Could you check a few things on this model? Use its own coordinates, in mm. A direction names the side the tool comes from. Coordinates: 2 decimals unless noted, no trailing zeros. Loops run counter-clockwise (first coordinate to the right, second up) from the corner with the lowest first, then second, coordinate; pieces in that order, holes last. Notation, with made-up numbers: M 2.25,72 L 9.25,72 A23 cw 9.25,92 Z; hole C 4,-29.5 d5. An arc over 180 degrees is marked long. Return JSON: item names as keys, results as strings. Group by question number.
from build123d import *

# Parameters (mm, degrees)
F0_W         = 64.9794517085
F0_H         = 80.3038775921
F1_DEPTH     = 44.704
F2_T         = -2.54
F3_R         = 24.241575959
F1_FACE1_W   = 44.704
F1_FACE1_H   = 80.3038775921
F4_DEPTH     = 10.668
F5_R         = 25.1594880742
F6_DEPTH     = 9.652
F7_W         = 6.6666891798
F7_H         = 7.7688368037
F8_DEPTH     = 37.846
F9_W         = 7.7688368037
F9_H         = 6.8424391291
F10_DEPTH    = 28.956
F11_W        = 7.8935802502
F11_H        = 7.7688368037
F12_DEPTH    = 25.4
F13_DEPTH    = 25.4
F15_DEPTH    = 34.798
F16_T1_DEPTH = 205.6075505485
F17_W        = 7.7688368037
F17_H        = 7.1335003994
F18_DEPTH    = 27.178


# Not quite as in the source:
# - a fillet or chamfer that OpenCascade refuses, or shapes differently, is made with other operations: its cross-section is extruded or revolved along the edge and cut away or added


with BuildPart() as f1:
    # F0 (on Front) → F1 (new body)
    with BuildSketch(Plane.XZ):
        with Locations((25.8230366744, -3.7049613893)):
            Rectangle(F0_W, F0_H)
    extrude(amount=F1_DEPTH)

    # F2
    f2_openings = [f1.faces().sort_by_distance(p)[0] for p in [
        (25.823037, -22.352, 36.446977),
        (25.823037, -44.704, -3.704961),
    ]]
    offset(amount=F2_T, openings=f2_openings)

    # F3 (on face) + F1_face1 (on face) → F4 (join)
    with BuildSketch(Plane.YZ.offset(58.3127625287)):
        with Locations((-22.6588118821, 0)):
            Circle(F3_R)
    with BuildSketch(Plane(origin=(-6.6666891798, -22.352, -3.7049613893), x_dir=(0, -1, 0), z_dir=(-1, 0, 0))):
        Rectangle(F1_FACE1_W, F1_FACE1_H)
    extrude(amount=F4_DEPTH, dir=(1, 0, 0))

    # F5 (on face) → F6 (join)
    with BuildSketch(Plane(origin=(-6.6666891798, 0, 0), x_dir=(0, -1, 0), z_dir=(-1, 0, 0))):
        with Locations((21.7208880931, 0)):
            Circle(F5_R)
    extrude(amount=F6_DEPTH)

    # F7 (on face) → F8 (join)
    with BuildSketch(Plane.XY.offset(36.4469774067)):
        with Locations((-3.3333445899, -17.414805945)):
            Rectangle(F7_W, F7_H)
    extrude(amount=F8_DEPTH)

    # F9 (on face) → F10 (join)
    with BuildSketch(Plane(origin=(-6.6666891798, 0, 0), x_dir=(0, -1, 0), z_dir=(-1, 0, 0))):
        with Locations((17.414805945, 70.8717578422)):
            Rectangle(F9_W, F9_H)
    extrude(amount=F10_DEPTH)

    # F11 (on face) → F12 (join)
    with BuildSketch(Plane.XY.offset(74.2929774067)):
        with Locations((-31.6758990547, -17.414805945)):
            Rectangle(F11_W, F11_H)
    extrude(amount=F12_DEPTH)

    # F13 (add): a face of the model
    f13_faces = [f1.faces().sort_by_distance(p)[0] for p in [
        (-31.6758990547, -17.414805945, 99.6929774067),
    ]]
    extrude(f13_faces, amount=F13_DEPTH)

    # F14 (on face) → F15 (join)
    with BuildSketch(Plane.XY.offset(36.4469774067)):
        Polygon((58.3127625287, -2.54), (58.3127625287, 0), (4.0013108202, 0), (4.0013108202, -2.54), (55.7727625287, -2.54), align=None)
    extrude(amount=F15_DEPTH)

    # F16: fillet of radius 181.5102324735 on 1 edges, made by hand

    # F16_s2 → F16_t1 (cut)
    with BuildSketch(Plane.YZ.offset(-71.6467385999)):
        with BuildLine():
            ThreePointArc((0, 71.2449774067), (-1.903885347, 56.1685767196), (-2.54, 40.9857576387))
            Line((-2.54, 40.9857576387), (-2.54, 71.2449774067))
            Line((-2.54, 71.2449774067), (0, 71.2449774067))
        make_face()
    extrude(amount=F16_T1_DEPTH, mode=Mode.SUBTRACT)

    # F17 (on face) → F18 (join)
    with BuildSketch(Plane.YZ.offset(-27.7291089296)):
        with Locations((-17.414805945, 121.5262272071)):
            Rectangle(F17_W, F17_H)
    extrude(amount=F18_DEPTH)


solid = f1.part
(1) Imagine slicing it at B-B, the plane z = 0. Write out the boundary of the cut face in (x, y), then the cut area to 3 significant figures.
(2) Imagine slicing it at C-C, the plane x = 51. Write out the boundary of the cut face in (y, z).
(3) For faces 1 (the face through (30, -23, -41.317)), 2 (the face through (-27.729, -17, 96)), 3 (the face through (-6.667, 1, 0)), which set-ups out of +Z, -Z, +X, -X, +Y, -Y let a thin tool reach every point of the face, with its end or its side?
(4) Imagine slicing it at D-D, the plane y = -25.5. Write out the boundary of the cut face in (x, z).
(5) Will these pins go through, and if not, where does the flat tip stop? P1, Ø3.5, axis at y = -18.5, z = 120, coming from the +X side; P2, Ø6, axis at x = 17.5, z = -7.5, coming from the -Y side; P3, Ø12, axis at y = -20, z = 12.5, coming from the -X side.
(6) We'd pull the mould along Z, two halves only. Please class faces 4 (the face through (25, -22, -43.857)), 5 (the face through (-16.319, -21, 0)), 6 (the face through (63.572, -41.896, -14.751)), 7 (the face through (-21, -17, 67.451)): +Z half, -Z half, draft (parallel to the pull), parting line (faces both ways), or undercut.
(7) If I drill on L1, parallel to X at y = -10, z = -24; L2, parallel to Z at x = -16, y = -14; L3, parallel to Z at x = -14, y = -18.5, over which ranges is the centre line in solid material (lowest first)? Write a range as [from, to].
(8) Imagine slicing it at A-A, the plane x = -8.5. Write out the boundary of the cut face in (y, z).
Checks:
{
 "1": {"outline": "M -16.32,-46.88 L -6.67,-46.88 L -6.67,-44.7 L 4,-44.7 L 4,-2.54 L 55.77,-2.54 L 55.77,-44.7 L 58.31,-44.7 L 58.31,-46.9 L 68.98,-46.9 L 68.98,1.58 L 58.31,1.58 L 58.31,0 L -6.67,0 L -6.67,3.44 L -16.32,3.44 Z", "area": "1,720 mm²"},
 "2": {"outline": "M -44.7,-43.86 L 0,-43.86 L 0,71.24 A181.51 ccw -2.54,40.99 L -2.54,-41.32 L -44.7,-41.32 Z"},
 "3": {"face 1": "+Z, -Y", "face 2": "+X, +Y, -Y", "face 3": "+Z, -Z, +Y"},
 "4": {"outline": "M -16.32,-24.87 L -6.67,-24.87 L -6.67,-43.86 L 58.31,-43.86 L 58.31,-24.07 L 68.98,-24.07 L 68.98,24.07 L 58.31,24.07 L 58.31,36.45 L 55.77,36.45 L 55.77,-41.32 L 4,-41.32 L 4,36.45 L -6.67,36.45 L -6.67,24.87 L -16.32,24.87 Z"},
 "5": {"P1": "x = -0.55", "P2": "y = -2.54", "P3": "x = -16.32"},
 "6": {"face 4": "-Z half", "face 5": "draft", "face 6": "parting line", "face 7": "undercut"},
 "7": {"L1": "[-6.67, 4], [55.77, 58.31]", "L2": "[-23.95, 23.95], [67.45, 74.29], [117.96, 125.09]", "L3": "[-24.95, 24.95], [67.45, 74.29], [117.96, 125.09]"},
 "8": {"outline": "C -21.72,0 d50.32; M -21.3,67.45 L -13.53,67.45 L -13.53,74.29 L -21.3,74.29 Z; M -21.3,117.96 L -13.53,117.96 L -13.53,125.09 L -21.3,125.09 Z"}
}
